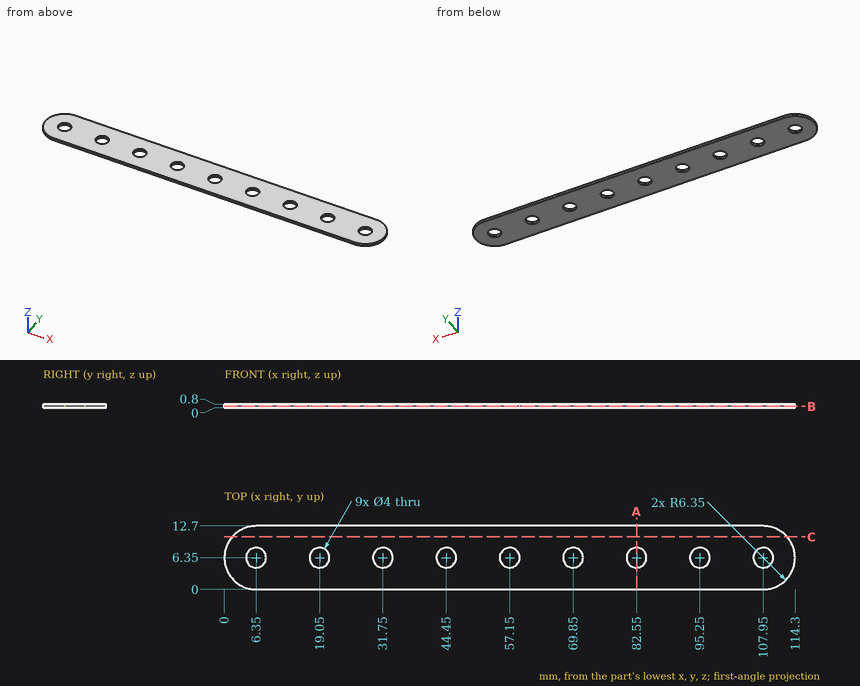
Geometry check sheet. Reference: drawing and pictorial views, mm from the part's lowest x, y, z. Give positions to 0.01 mm unless a question says otherwise; leave off trailing zeros. Order: outer loops, then holes, each group sorted by start corner. A loop starts at its lowest first (then second) coordinate and runs counter-clockwise, first axis right, second up. Notation, with made-up numbers: M 68,-39.5 L 120,-39.5 A11 ccw 120,-34.5 Z; hole C 58,30.5 d4. An arc over 180 degrees is marked long. Use one line per item in the form item = value. Start each with the question number.
Q1. Section check B-B (z = 0.3). Count the separate pieces of the cut face and the enclosed holes in it, then the cut area to 3 significant figures.
Q2. Section check A-A (x = 82.55). Enter the section's corners in (y, z).
Q3. Section check C-C (y = 10.5). Enter the section's corners in (x, z).
Q4. Scan lines: line 1 along Y through (x, z) = (107.95, 0.35); line 2 along Y through (x, z) = (5.5, 0.6); line 3 along X through (y, z) = (1.5, 0.75). Record each from-to range of solid material in increasing order. Write a range as [from, to].
Evaluation:
q1.separate_pieces = 1
q1.enclosed_holes = 9
q1.area = 1,300 mm2
q2.outline = M 0,0 L 4.35,0 L 4.35,0.8 L 0,0.8 Z; M 8.35,0 L 12.7,0 L 12.7,0.8 L 8.35,0.8 Z
q3.outline = M 1.54,0 L 112.76,0 L 112.76,0.8 L 1.54,0.8 Z
q4.line_1 = [0, 4.35], [8.35, 12.7]
q4.line_2 = [0.06, 4.54], [8.16, 12.64]
q4.line_3 = [2.25, 112.05]
